Read the model definition and answer for the solid it produces. Units are mm, in the model's axes. A direction names the side the tool comes from. Round coordinates to 2 decimals unless told otherwise and drop trailing zeros. Loops run counter-clockwise (first coordinate to the right, second up) from the corner with the lowest first, then second, coordinate; pieces in that order, holes last. Notation, with made-up numbers: (18, -13.5) - (59, -13.5) arc R26 ccw to (59, 13.5) - close; hole circle Ø2 at (80.25, 10.25). An arc over 180 degrees is marked (long way). Use CSV: the item, a comma, the result in double quotes. Start each with the question number.
1. A tool of negligible diameter and unlimited length cuts with its end or side. For faces 1 (the flat face through (232, 13, 3.175)), 2 (the flat face through (232, 25.4, 13)), from which of +Z, -Z, +X, -X, +Y, -Y can it reach the whole face along a straight path? Write none if from no direction.
2. Consider line 1 along Y through (x, z) = (331.5, 14) (3 decimals); line 2 along Y through (x, z) = (419.1, 23.2). Determine where each line is inside the solid, lowest interval first.
3. Determine the mould class of faces 3 (the flat face through (0, 2, 13)), 4 (the flat face through (232, 13, 22.225)), 5 (the flat face through (225, 0, 13)) for opening direction Y: +Y half, -Y half, draft (parallel to the pull), parting line (faces both ways), or undercut.
4. Find section A-A (x = 375.5). Give the vertices of the cut face in (y, z) (3 decimals).
5. Given pin 1 Ø2.5 at (x, y) = (38.1, 12.7) entering from -Z; pin 2 Ø4 at (y, z) = (3.5, 17) entering from -X, each flat-ended and moving along its own axis, determine where each tip first touches the part or whether it passes through.
Autodesk Inventor part; units mm, degrees
ref_plane "YZ Plane" through (0, 0, 0) normal (1, 0, 0) x (0, 1, 0)
ref_plane "XZ Plane" through (0, 0, 0) normal (0, 1, 0) x (-1, 0, 0)
ref_plane "XY Plane" through (0, 0, 0) normal (0, 0, 1) x (1, 0, 0)
sketch "Sketch1" plane through (0, 0, 0) normal (0, 0, 1) x (1, 0, 0)
  line L0 (0, 0) -> (660.4, 0)
  line L1 (660.4, 0) -> (660.4, 25.4)
  line L2 (660.4, 25.4) -> (0, 25.4)
  line L3 (0, 25.4) -> (0, 0)
  dimension "d0" = 660.4
  dimension "d1" = 25.4
extrude "Extrusion1" add sketch "Sketch1" along normal blind 25.4
sketch "Sketch2" plane through (0, 25.4, 0) normal (0, 1, 0) x (1, 0, 0)
  circle A0 centre (9.5046, -12.7) radius 1.9685
  line L0 (660.4, 0) -> (0, 0)
  circle A1 centre (34.9046, -12.7) radius 1.9685
  circle A2 centre (60.3046, -12.7) radius 1.9685
  circle A3 centre (85.7046, -12.7) radius 1.9685
  circle A4 centre (111.1046, -12.7) radius 1.9685
  circle A5 centre (136.5046, -12.7) radius 1.9685
  circle A6 centre (161.9046, -12.7) radius 1.9685
  circle A7 centre (187.3046, -12.7) radius 1.9685
  circle A8 centre (212.7046, -12.7) radius 1.9685
  circle A9 centre (238.1046, -12.7) radius 1.9685
  circle A10 centre (263.5046, -12.7) radius 1.9685
  circle A11 centre (288.9046, -12.7) radius 1.9685
  circle A12 centre (314.3046, -12.7) radius 1.9685
  circle A13 centre (339.7046, -12.7) radius 1.9685
  circle A14 centre (365.1046, -12.7) radius 1.9685
  circle A15 centre (390.5046, -12.7) radius 1.9685
  circle A16 centre (415.9046, -12.7) radius 1.9685
  circle A17 centre (441.3046, -12.7) radius 1.9685
  circle A18 centre (466.7046, -12.7) radius 1.9685
  circle A19 centre (492.1046, -12.7) radius 1.9685
  circle A20 centre (517.5046, -12.7) radius 1.9685
  circle A21 centre (542.9046, -12.7) radius 1.9685
  circle A22 centre (568.3046, -12.7) radius 1.9685
  circle A23 centre (593.7046, -12.7) radius 1.9685
  circle A24 centre (619.1046, -12.7) radius 1.9685
  circle A25 centre (644.5046, -12.7) radius 1.9685
  dimension "d4" = 3.937
  dimension "d5" = 12.7
  dimension "d8" = 25.4
extrude "Extrusion2" cut sketch "Sketch2" against normal blind 25.4
sketch "Sketch3" plane through (660.4, 0, 0) normal (1, 0, 0) x (0, 0, -1)
  line L0 (-3.175, 22.225) -> (-22.225, 22.225)
  line L1 (-22.225, 22.225) -> (-22.225, 3.175)
  line L2 (-22.225, 3.175) -> (-3.175, 3.175)
  line L3 (-3.175, 3.175) -> (-3.175, 22.225)
  line L4 (0, 25.4) -> (-25.4, 25.4)
  line L5 (0, 0) -> (0, 25.4)
  line L6 (0, 0) -> (-25.4, 0)
  line L7 (-25.4, 0) -> (-25.4, 25.4)
  dimension "d15" = 3.175
  dimension "d16" = 3.175
  dimension "d17" = 3.175
  dimension "d18" = 3.175
extrude "Extrusion3" cut sketch "Sketch3" against normal blind 660.4 contours L3 L2 L1 L0
sketch "Sketch4" plane through (0, 0, 0) normal (0, 0, -1) x (-1, 0, 0)
  circle A0 centre (-12.7, 12.7) radius 1.9685
  line L0 (-660.4, 25.4) -> (0, 25.4)
  line L1 (0, 25.4) -> (0, 0)
  circle A1 centre (-38.1, 12.7) radius 1.9685
  circle A2 centre (-63.5, 12.7) radius 1.9685
  circle A3 centre (-88.9, 12.7) radius 1.9685
  circle A4 centre (-114.3, 12.7) radius 1.9685
  circle A5 centre (-139.7, 12.7) radius 1.9685
  circle A6 centre (-165.1, 12.7) radius 1.9685
  circle A7 centre (-190.5, 12.7) radius 1.9685
  circle A8 centre (-215.9, 12.7) radius 1.9685
  circle A9 centre (-241.3, 12.7) radius 1.9685
  circle A10 centre (-266.7, 12.7) radius 1.9685
  circle A11 centre (-292.1, 12.7) radius 1.9685
  circle A12 centre (-317.5, 12.7) radius 1.9685
  circle A13 centre (-342.9, 12.7) radius 1.9685
  circle A14 centre (-368.3, 12.7) radius 1.9685
  circle A15 centre (-393.7, 12.7) radius 1.9685
  circle A16 centre (-419.1, 12.7) radius 1.9685
  circle A17 centre (-444.5, 12.7) radius 1.9685
  circle A18 centre (-469.9, 12.7) radius 1.9685
  circle A19 centre (-495.3, 12.7) radius 1.9685
  circle A20 centre (-520.7, 12.7) radius 1.9685
  circle A21 centre (-546.1, 12.7) radius 1.9685
  circle A22 centre (-571.5, 12.7) radius 1.9685
  circle A23 centre (-596.9, 12.7) radius 1.9685
  circle A24 centre (-622.3, 12.7) radius 1.9685
  circle A25 centre (-647.7, 12.7) radius 1.9685
  dimension "d21" = 3.937
  dimension "d22" = 12.7
  dimension "d23" = 12.7
  dimension "d26" = 25.4
extrude "Extrusion4" cut sketch "Sketch4" against normal blind 25.4
sketch "Sketch5" plane through (660.4, 0, 0) normal (1, 0, 0) x (0, 0, -1)
  line L0 (0, 25.4) -> (-25.4, 25.4)
  line L1 (0, 0) -> (-25.4, 0)
  line L2 (-25.4, 25.4) -> (0, 25.4)
  line L3 (0, 25.4) -> (0, 0)
  line L4 (0, 0) -> (-25.4, 0)
  line L5 (-25.4, 0) -> (-25.4, 25.4)
extrude "Extrusion5" cut sketch "Sketch5" against normal blind 203.2
properties part number "kermit frame 4"
Filled sheet:
1,face 1,"+X, -X"
1,face 2,"+Z, -Z, +X, -X, +Y"
2,line 1,"y = 0 to 3.175, 22.225 to 25.4"
2,line 2,"y = 0 to 10.73, 14.67 to 25.4"
3,face 3,"draft"
3,face 4,"undercut"
3,face 5,"-Y half"
4,outline,"(0, 0) - (25.4, 0) - (25.4, 25.4) - (0, 25.4) - close; hole (3.175, 3.175) - (22.225, 3.175) - (22.225, 22.225) - (3.175, 22.225) - close"
5,pin 1,"passes through"
5,pin 2,"stops at x = 0"
